Can you work these out from the model? Positions are in its coordinate system, mm. A direction names the side the tool comes from. Give positions to 0.01 mm unless a question says otherwise; leave off trailing zeros. Loops run counter-clockwise (first coordinate to the right, second up) from the corner with the lowest first, then second, coordinate; pieces in that order, holes last. Notation, with made-up numbers: M -15.5,28 L -3.5,28 A22 ccw -3.5,64 Z; hole C 75,-36.75 d1. An arc over 180 degrees is marked long. Use CSV: the item, a comma, the result in double quotes.
from build123d import *

# Parameters (mm, degrees)
F1_DEPTH = 80
F3_DEPTH = 42.701
F4_R     = 1.3
F4_R_2   = 1.35
F5_DEPTH = 8.001


with BuildPart() as f1:
    # F0 (on Right) → F1 (new body)
    with BuildSketch(Plane.YZ):
        Polygon((0, 35), (0, 0), (42.7, 0), (42.7, 8), (2.7, 8), (2.7, 35), align=None)
    extrude(amount=F1_DEPTH)

    # F2 (on face) → F3 (cut, through all)
    with BuildSketch(Plane.XZ):
        with BuildLine():
            Line((13.388215, 28.4), (6.611785, 28.4))
            ThreePointArc((6.611785, 28.4), (10, 20.2), (13.388215, 28.4))
        make_face()
        with BuildLine():
            Line((33.388215, 28.4), (26.611785, 28.4))
            ThreePointArc((26.611785, 28.4), (30, 20.2), (33.388215, 28.4))
        make_face()
        with BuildLine():
            Line((53.388215, 28.4), (46.611785, 28.4))
            ThreePointArc((46.611785, 28.4), (50, 20.2), (53.388215, 28.4))
        make_face()
        with BuildLine():
            Line((73.388215, 28.4), (66.611785, 28.4))
            ThreePointArc((66.611785, 28.4), (70, 20.2), (73.388215, 28.4))
        make_face()
    extrude(amount=-F3_DEPTH, mode=Mode.SUBTRACT)

    # F4 (on face) → F5 (cut, through all)
    with BuildSketch(Plane.XY.offset(8)):
        with Locations((5, 37.7)):
            Circle(F4_R)
        with Locations((75, 37.7)):
            Circle(F4_R)
        with Locations((14.6, 17.7)):
            Circle(F4_R_2)
        with Locations((27.3, 17.7)):
            Circle(F4_R_2)
        with Locations((1.9, 17.7)):
            Circle(F4_R_2)
        with Locations((40, 17.7)):
            Circle(F4_R_2)
        with Locations((52.7, 17.7)):
            Circle(F4_R_2)
        with Locations((65.4, 17.7)):
            Circle(F4_R_2)
        with Locations((78.1, 17.7)):
            Circle(F4_R_2)
    extrude(amount=-F5_DEPTH, mode=Mode.SUBTRACT)


solid = f1.part
Q1. I want a section at D-D, the plane x = 17. Please give me the cut outline in (y, z).
Model answer:
outline,"M 0,0 L 42.7,0 L 42.7,8 L 2.7,8 L 2.7,35 L 0,35 Z"
Q2. If we mould it in two halves opening along X, with no side actions, what happens to faces 4 (the cylindrical face through (79.388, 18.106, 4.056)), 5 (the flat face through (80, 17, 7)), 6 (the flat face through (39, 2.7, 21))? For each: released by +X, released by -X, zero draft, split by the parting line, or undercut.
Model answer:
face 4,"undercut"
face 5,"released by +X"
face 6,"zero draft"
Q3. Please list where these lines run through material, in increasing order: L1, parallel to Z at x = 70, y = 1; L2, parallel to Y at x = 19.5, z = 25; L3, parallel to Z at x = 24.5, y = 9.5. Write a range as from..to.
Model answer:
L1,"0..20.2, 28.4..35"
L2,"0..2.7"
L3,"0..8"
Q4. I want a section at B-B, the plane y = 37.7. Please give me the cut outline in (x, z).
Model answer:
outline,"M 0,0 L 3.7,0 L 3.7,8 L 0,8 Z; M 6.3,0 L 73.7,0 L 73.7,8 L 6.3,8 Z; M 76.3,0 L 80,0 L 80,8 L 76.3,8 Z"
Q5. I'm going to push flat-ended pins straight in: P1, Ø1.5, axis at x = 39.5, z = 9, coming from the +Y side; P2, Ø3.5, axis at x = 75, y = 37.7, coming from the +Z side. Where does each tip first touch, or does it pass through?
Model answer:
P1,"y = 2.7"
P2,"z = 8"
Q6. I want a section at C-C, the plane z = 21. Please give me the cut outline in (x, y).
Model answer:
outline,"M 0,0 L 7.35,0 L 7.35,2.7 L 0,2.7 Z; M 12.65,0 L 27.35,0 L 27.35,2.7 L 12.65,2.7 Z; M 32.65,0 L 47.35,0 L 47.35,2.7 L 32.65,2.7 Z; M 52.65,0 L 67.35,0 L 67.35,2.7 L 52.65,2.7 Z; M 72.65,0 L 80,0 L 80,2.7 L 72.65,2.7 Z"
Q7. I want a section at A-A, the plane x = 30. Please give me the cut outline in (y, z), then the cut area to 3 significant figures.
Model answer:
outline,"M 0,0 L 42.7,0 L 42.7,8 L 2.7,8 L 2.7,20.2 L 0,20.2 Z; M 0,28.4 L 2.7,28.4 L 2.7,35 L 0,35 Z"
area,"392 mm2"
Q8. For faces 1 (the cylindrical face through (75.699, 38.796, 4.056)), 2 (the flat face through (39, 23, 8)), 3 (the flat face through (70, 1, 28.4)), which set-ups out of +Z, -Z, +X, -X, +Y, -Y let a thin tool reach every point of the face, with its end or its side?
Model answer:
face 1,"+Z, -Z"
face 2,"+Z, +X, -X, +Y"
face 3,"+Y, -Y"
